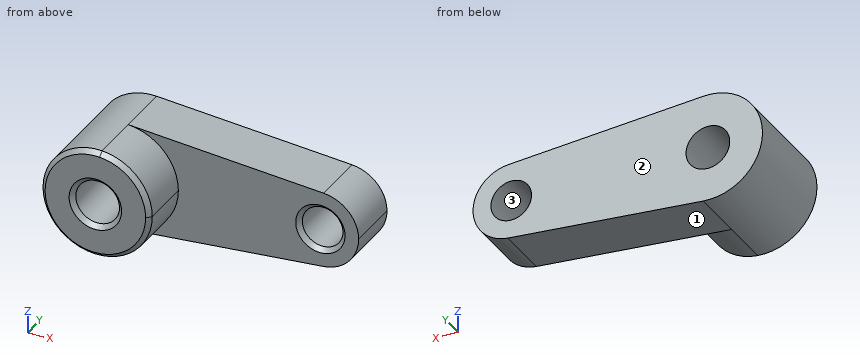
```python
from build123d import *

# Parameters (mm, degrees)
F0_R     = 10
F0_R_2   = 9.297585
F1_DEPTH = 25
F2_DEPTH = 50
F3_SIZE  = 2


with BuildPart() as f1:
    # F0 (on Front) → F1 (new body)
    with BuildSketch(Plane.XZ):
        with BuildLine():
            ThreePointArc((2.083333, -24.913043), (18.399502, -16.92508), (25, 0))
            ThreePointArc((25, 0), (18.399502, 16.92508), (2.083333, 24.913043))
            ThreePointArc((2.083333, 24.913043), (-25, 0), (2.083333, -24.913043))
        make_face()
        Circle(F0_R, mode=Mode.SUBTRACT)
        with BuildLine():
            ThreePointArc((2.083333, 24.913043), (18.399502, 16.92508), (25, 0))
            ThreePointArc((25, 0), (18.399502, -16.92508), (2.083333, -24.913043))
            Line((2.083333, -24.913043), (91.458333, -17.43913))
            ThreePointArc((91.458333, -17.43913), (72.5, 0), (91.458333, 17.43913))
            Line((91.458333, 17.43913), (2.083333, 24.913043))
        make_face()
        with BuildLine():
            ThreePointArc((107.5, 0), (102.879651, 11.847556), (91.458333, 17.43913))
            ThreePointArc((91.458333, 17.43913), (72.5, 0), (91.458333, -17.43913))
            ThreePointArc((91.458333, -17.43913), (102.879651, -11.847556), (107.5, 0))
        make_face()
        with Locations((90, 0)):
            Circle(F0_R_2, mode=Mode.SUBTRACT)
    extrude(amount=F1_DEPTH)

    # F0 (on Front) → F2 (join)
    with BuildSketch(Plane.XZ):
        with BuildLine():
            ThreePointArc((2.083333, -24.913043), (18.399502, -16.92508), (25, 0))
            ThreePointArc((25, 0), (18.399502, 16.92508), (2.083333, 24.913043))
            ThreePointArc((2.083333, 24.913043), (-25, 0), (2.083333, -24.913043))
        make_face()
        Circle(F0_R, mode=Mode.SUBTRACT)
    extrude(amount=F2_DEPTH)

    # F3
    f3_edges = [f1.edges().sort_by_distance(p)[0] for p in [
        (80.702415, -25, 0),
        (-10, -50, 0),
        (-2.083333, -50, 24.913043),
    ]]
    chamfer(f3_edges, length=F3_SIZE)


solid = f1.part
```
Here's how the part is built. I have some questions about the finished solid (model axes, mm). Face numbers are marked on the shaded views. Coordinates: 2 decimals unless noted, no trailing zeros. Loops run counter-clockwise (first coordinate to the right, second up) from the corner with the lowest first, then second, coordinate; pieces in that order, holes last. Notation, with made-up numbers: (10, 54.25) - (69, 54.25) arc R18 ccw to (69, 63.25) - close; hole circle Ø6 at (74, 48). An arc over 180 degrees is marked (long way). Return JSON: item names as keys, results as strings. Group by question number.
Item 1: If we section it at B-B on y = -14.5: Write out the boundary of the cut face in (x, z).
Item 2: Will these pins go through, and if not, where does the flat tip stop? P1, Ø10, axis at x = 13, y = -37.5, coming from the +Z side; P2, Ø1, axis at x = 29, y = -7.5, coming from the +Z side; P3, Ø8, axis at x = 39, z = -17.5, coming from the -Y side.
Item 3: If we section it at A-A on x = 0: Write out the boundary of the cut face in (y, z).
Item 4: I need wall thicknesses on line 1 (Z direction, x = 0, y = -33); line 2 (X direction, y = -4.5, z = -1); line 3 (Y direction, x = 52.5, z = -13). Which ranges of each line are inside material? Lowest first, please. Write a range as from..to.
Item 5: We'd pull the mould along Z, two halves only. Please class the marked faces 1, 2 and 3: +Z half, -Z half, draft (parallel to the pull), parting line (faces both ways), or undercut.
Item 6: If we section it at D-D on z = 4: State how many separate pieces and enclosed holes the cut face has, and give its area (3 significant figures).
Item 7: If we section it at C-C on y = -36.5: Write out the boundary of the cut face in (x, z), and give its area (3 significant figures).
Calculated:
{
 "1": {"outline": "(2.08, -24.91) - (91.46, -17.44) arc R17.5 ccw to (91.46, 17.44) - (2.08, 24.91) arc R25 ccw (long way) to start; hole circle Ø20 at (0, 0); hole circle Ø18.6 at (90, 0)"},
 "2": {"P1": "stops at z = 23.69", "P2": "stops at z = 22.7", "P3": "stops at y = -25"},
 "3": {"outline": "(-50, -23) - (-48, -25) - (0, -25) - (0, -10) - (-48, -10) - (-50, -12) - close; (-50, 12) - (-48, 10) - (0, 10) - (0, 25) - (-48, 25) - (-50, 23) - close"},
 "4": {"line 1": "z = -25..-10, 10..25", "line 2": "x = -24.98..-9.95, 9.95..80.76, 99.24..107.47", "line 3": "y = -25..0"},
 "5": {"face 1": "-Z half", "face 2": "draft", "face 3": "undercut"},
 "6": {"separate pieces": "3", "enclosed holes": "0", "area": "3,180 mm^2"},
 "7": {"outline": "(2.08, -24.91) arc R25 ccw to (25, 0) arc R25 ccw to (2.08, 24.91) arc R25 ccw (long way) to start; hole circle Ø20 at (0, 0)", "area": "1,650 mm^2"}
}
